from build123d import *

# Parameters (mm, degrees)
BOSS_EXTRUDE1_DEPTH = 10.16
SKETCH2_R           = 2.54
CUT_EXTRUDE1_DEPTH  = 33.773906903


with BuildPart() as part:
    # Sketch1 → Boss-Extrude1 (new body)
    with BuildSketch(Plane.XY):
        with BuildLine():
            Line((-11.415908645, -15.267119982), (-30.465908645, -15.267119982))
            Line((-30.465908645, -15.267119982), (-30.465908645, -21.671319081))
            Line((-30.465908645, -21.671319081), (30.494091355, -21.671319081))
            Line((30.494091355, -21.671319081), (30.494091355, -15.267119982))
            Line((30.494091355, -15.267119982), (11.444091355, -15.267119982))
            ThreePointArc((11.444091355, -15.267119982), (0.014091355, -19.077119982), (-11.415908645, -15.267119982))
        make_face()
    extrude(amount=BOSS_EXTRUDE1_DEPTH)

    # Sketch2 → Cut-Extrude1 (cut, through all)
    with BuildSketch(Plane(origin=(0, -15.267119982, 0), x_dir=(1, 0, 0), z_dir=(0, 1, 0))):
        with Locations(Location((-25.392954322, -5.08, 0), (0, 0, 180))):
            Circle(SKETCH2_R)
        with Locations((25.406947958, -5.00954336)):
            Circle(SKETCH2_R)
    extrude(amount=-CUT_EXTRUDE1_DEPTH, mode=Mode.SUBTRACT)


solid = part.part
Build history of the part. All positions in model axes, mm. Give positions to 0.01 mm unless a question says otherwise; leave off trailing zeros. Loops run counter-clockwise (first coordinate to the right, second up) from the corner with the lowest first, then second, coordinate; pieces in that order, holes last. Notation, with made-up numbers: (-21, 12.25) -> (-17, 12.25) arc R30 ccw to (-17, 44.25) -> close; hole circle Ø10 at (81.5, 31). An arc over 180 degrees is marked (long way). Answer in a Markdown table with one row per item.
Item 1: Mould opens along Z. For faces 1 (the cylindrical face through (24.9, -18.4, 7.5)), 2 (the cylindrical face through (-23.38, -18.42, 3.53)), 3 (the flat face through (0, -20, 10.16)), 4 (the flat face through (-21, -15.267, 5)) say: pulls with the +Z half, pulls with the -Z half, needs draft (parallel to the pull), parting line crosses it, or undercut.
Findings below:
| item | result |
|---|---|
| face 1 | undercut |
| face 2 | undercut |
| face 3 | pulls with the +Z half |
| face 4 | needs draft |
Item 2: Slice it at D-D on x = 8.5. Write the cut outline in (y, z).
Findings below:
| item | result |
|---|---|
| outline | (-21.67, 0) -> (-17.08, 0) -> (-17.08, 10.16) -> (-21.67, 10.16) -> close |
Item 3: Probe line 1 along X through (y, z) = (-20, 5.5); line 2 along X through (y, z) = (-16.5, 5.75); line 3 along X through (y, z) = (-16.25, 5.25). List the from-to ranges inside material, lowest first. Write a range as [from, to].
Findings below:
| item | result |
|---|---|
| line 1 | x = [-30.47, -27.9], [-22.89, 22.91], [27.9, 30.49] |
| line 2 | x = [-30.47, -27.84], [-22.94, -9.55], [9.58, 22.98], [27.84, 30.49] |
| line 3 | x = [-30.47, -27.93], [-22.86, -9.97], [10, 22.88], [27.94, 30.49] |
Item 4: Slice it at A-A on y = -18.5. Write the cut outline in (x, z), plus the area to 3 significant figures.
Findings below:
| item | result |
|---|---|
| outline | (-30.47, 0) -> (-4.64, 0) -> (-4.64, 10.16) -> (-30.47, 10.16) -> close; (4.67, 0) -> (30.49, 0) -> (30.49, 10.16) -> (4.67, 10.16) -> close; hole circle Ø5.08 at (-25.39, 5.08); hole circle Ø5.08 at (25.41, 5.01) |
| area | 484 mm² |
Item 5: Slice it at B-B on z = 4.25. Write the cut outline in (x, y), plus the area to 3 significant figures.
Findings below:
| item | result |
|---|---|
| outline | (-30.47, -21.67) -> (-27.79, -21.67) -> (-27.79, -15.27) -> (-30.47, -15.27) -> close; (-22.99, -21.67) -> (22.98, -21.67) -> (22.98, -15.27) -> (11.44, -15.27) arc R19.05 cw to (-11.42, -15.27) -> (-22.99, -15.27) -> close; (27.83, -21.67) -> (30.49, -21.67) -> (30.49, -15.27) -> (27.83, -15.27) -> close |
| area | 269 mm² |
Item 6: Flat gauge pin, fed straight in: P1, Ø1.5, axis at x = -5, z = 8, coming from the +Y side. Where does the tip first touch, or does it go through?
Findings below:
| item | result |
|---|---|
| P1 | stops at y = -18.18 |
Item 7: Slice it at C-C on z = 0.75. Write the cut outline in (x, y).
Findings below:
| item | result |
|---|---|
| outline | (-30.47, -21.67) -> (30.49, -21.67) -> (30.49, -15.27) -> (11.44, -15.27) arc R19.05 cw to (-11.42, -15.27) -> (-30.47, -15.27) -> close |
